Here's how the part is built. I have some questions about the finished solid (model axes, mm). Face numbers are marked on the shaded views. Round coordinates to 2 decimals unless told otherwise and drop trailing zeros. Use one line per item in the form item = value. Start each with the question number.
```python
from build123d import *

# Parameters (mm, degrees)
SKETCH1_W           = 1190
SKETCH1_H           = 635
BOSS_EXTRUDE1_DEPTH = 5
SKETCH2_R           = 1.2
SKETCH2_R_2         = 1.5
CUT_EXTRUDE1_DEPTH  = 10
CUT_EXTRUDE2_START  = -10
SKETCH4_R           = 1.5
CUT_EXTRUDE2_DEPTH  = 10
SKETCH5_R           = 1.2
CUT_EXTRUDE3_DEPTH  = 10


with BuildPart() as part:
    # Sketch1 → Boss-Extrude1 (new body)
    with BuildSketch(Plane.XY):
        Rectangle(SKETCH1_W, SKETCH1_H)
    extrude(amount=BOSS_EXTRUDE1_DEPTH)

    # Sketch2 → Cut-Extrude1 (cut)
    with BuildSketch(Plane.ZY.offset(595)):
        with Locations((2.5, -320)):
            Circle(SKETCH2_R)
        with Locations((2.5, 302.5)):
            Circle(SKETCH2_R_2)
    extrude(amount=-CUT_EXTRUDE1_DEPTH, mode=Mode.SUBTRACT)

    # Sketch4 → Cut-Extrude2 (cut)
    with BuildSketch(Plane(origin=(595, 0, 0), x_dir=(0, 0, -1), z_dir=(1, 0, 0)).offset(CUT_EXTRUDE2_START)):
        with Locations(Location((-2.5, 302.5, 0), (0, 0, 180))):
            Circle(SKETCH4_R)
        with Locations((-2.5, -307.5)):
            Circle(SKETCH4_R)
    extrude(amount=CUT_EXTRUDE2_DEPTH, mode=Mode.SUBTRACT)

    # Sketch5 → Cut-Extrude3 (cut)
    with BuildSketch(Plane(origin=(595, 0, 0), x_dir=(0, 0, -1), z_dir=(1, 0, 0))):
        with Locations((-2.5, 315)):
            Circle(SKETCH5_R)
    extrude(amount=-CUT_EXTRUDE3_DEPTH, mode=Mode.SUBTRACT)


solid = part.part
```
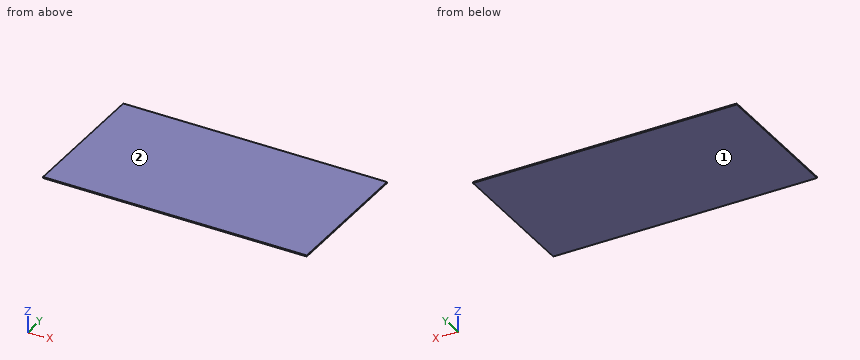
1) If I drill on line 1 (Y direction, x = 591.75, z = 2.5); line 2 (Z direction, x = 587, y = -307.5); line 3 (Y direction, x = -591.75, z = 2.5), over which ranges is the centre line in solid material (lowest first)?
2) If we mould it in two halves opening along Z, with no side actions, what happens to the marked faces 1 and 2? For each: +Z half, -Z half, draft (parallel to the pull), parting line (faces both ways), or undercut.
3) Will this pin go through, and if not, where does the flat tip stop? pin 1 Ø2.5 at (y, z) = (302.5, 2.5) entering from +X.
Completed:
q1.line_1 = -317.5 to -309, -306 to 301, 304 to 313.8, 316.2 to 317.5
q1.line_2 = 0 to 1, 4 to 5
q1.line_3 = -317.5 to 301, 304 to 317.5
q2.face_1 = -Z half
q2.face_2 = +Z half
q3.pin_1 = 585
